```python
from build123d import *

# Parameters (mm, degrees)
SKETCH1_R           = 75
BOSS_EXTRUDE1_DEPTH = 6.35
SKETCH45_R          = 22.1615
SKETCH45_R_2        = 2.0193
CUT_EXTRUDE36_DEPTH = 107.255929246
FILLET2_R           = 10.16


with BuildPart() as part:
    # Sketch1 → Boss-Extrude1 (new body)
    with BuildSketch(Plane(origin=(0, 0, 0), x_dir=(1, 0, 0), z_dir=(0, 1, 0))):
        with Locations(Location((0, 0, 0), (0, 0, 270))):
            Circle(SKETCH1_R)
    extrude(amount=BOSS_EXTRUDE1_DEPTH)

    # Sketch45 → Cut-Extrude36 (cut, through all)
    with BuildSketch(Plane(origin=(0, 6.35, 0), x_dir=(1, 0, 0), z_dir=(0, 1, 0))):
        with Locations(Location((0, 0, 0), (0, 0, 270))):
            Circle(SKETCH45_R)
        with Locations(Location((0, 33.02, 0), (0, 0, 270))):
            Circle(SKETCH45_R_2)
        with Locations(Location((-33.02, 0, 0), (0, 0, 270))):
            Circle(SKETCH45_R_2)
        with Locations(Location((0, -33.02, 0), (0, 0, 270))):
            Circle(SKETCH45_R_2)
        with Locations(Location((33.02, 0, 0), (0, 0, 270))):
            Circle(SKETCH45_R_2)
        with Locations(Location((-25.4, 25.4, 0), (0, 0, 270))):
            Circle(SKETCH45_R_2)
        with BuildLine():
            Line((-32.276051224, 28.683948776), (-54.798637954, 51.206535505))
            ThreePointArc((-54.798637954, 51.206535505), (-54.798637954, 54.798637954), (-51.206535505, 54.798637954))
            Line((-51.206535505, 54.798637954), (-28.683948776, 32.276051224))
            ThreePointArc((-28.683948776, 32.276051224), (-28.683948776, 28.683948776), (-32.276051224, 28.683948776))
        make_face()
        with BuildLine():
            Line((-28.683948776, -32.276051224), (-51.206535505, -54.798637954))
            ThreePointArc((-51.206535505, -54.798637954), (-54.798637954, -54.798637954), (-54.798637954, -51.206535505))
            Line((-54.798637954, -51.206535505), (-32.276051224, -28.683948776))
            ThreePointArc((-32.276051224, -28.683948776), (-28.683948776, -28.683948776), (-28.683948776, -32.276051224))
        make_face()
    extrude(amount=-CUT_EXTRUDE36_DEPTH, mode=Mode.SUBTRACT)

    # Fillet2
    fillet2_edges = [part.edges().sort_by_distance(p)[0] for p in [
        (-51.206535505, 3.175, 54.798637954),
        (-54.798637954, 3.175, 51.206535505),
        (-54.798637954, 3.175, -51.206535505),
        (-51.206535505, 3.175, -54.798637954),
    ]]
    fillet(fillet2_edges, radius=FILLET2_R)


solid = part.part
```
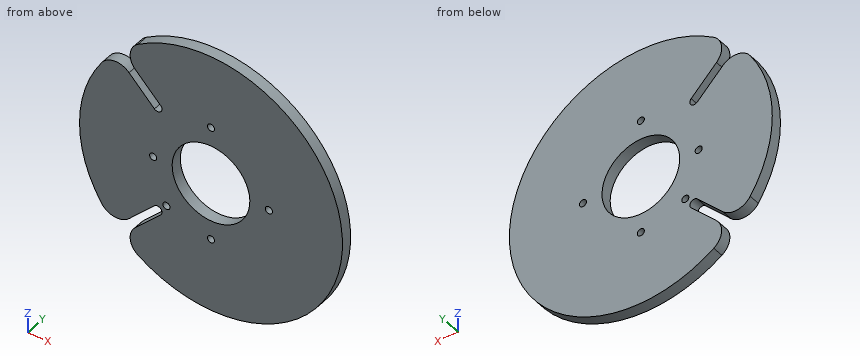
For this review, take the finished solid that the model builds, in its own axes (mm). Give positions to 0.01 mm unless a question says otherwise; leave off trailing zeros. Write each loop counter-clockwise with the first axis right and the second up, starting at its lowest first coordinate (ties: lowest second). Pieces come first, ordered by that corner, then holes. Notation, with made-up numbers: M 26,62 L 60,62 A14 ccw 60,80 Z; hole C 26,89.25 d2. An arc over 180 degrees is marked long. One line per item, written item: value.
1) Take a section at C-C, the plane z = 0. Write out the cut boundary in (x, y), then the cut area to 3 significant figures.
Results are:
outline: M -75,0 L -35.04,0 L -35.04,6.35 L -75,6.35 Z; M -31,0 L -22.16,0 L -22.16,6.35 L -31,6.35 Z; M 22.16,0 L 31,0 L 31,6.35 L 22.16,6.35 Z; M 35.04,0 L 75,0 L 75,6.35 L 35.04,6.35 Z
area: 620 mm²
2) Take a section at A-A, the plane y = 3. Write out the cut boundary in (x, z), then the cut area to 3 significant figures.
Results are:
outline: M -62.39,-41.62 A10.16 ccw -46.76,-43.16 L -32.28,-28.68 A2.54 cw -28.68,-32.28 L -43.16,-46.76 A10.16 ccw -41.62,-62.39 A75 ccw long -41.62,62.39 A10.16 ccw -43.16,46.76 L -28.68,32.28 A2.54 cw -32.28,28.68 L -46.76,43.16 A10.16 ccw -62.39,41.62 A75 ccw Z; hole C -33.02,0 d4.04; hole C -25.4,-25.4 d4.04; hole C 0,0 d44.32; hole C 0,-33.02 d4.04; hole C 0,33.02 d4.04; hole C 33.02,0 d4.04
area: 15,600 mm²
3) Take a section at D-D, the plane x = -25.4. Write out the cut boundary in (y, z), then the cut area to 3 significant figures.
Results are:
outline: M 0,-70.57 L 6.35,-70.57 L 6.35,-27.42 L 0,-27.42 Z; M 0,-23.38 L 6.35,-23.38 L 6.35,70.57 L 0,70.57 Z
area: 871 mm²
4) Take a section at B-B, the plane x = 17.5. Write out the cut boundary in (y, z).
Results are:
outline: M 0,-72.93 L 6.35,-72.93 L 6.35,-13.6 L 0,-13.6 Z; M 0,13.6 L 6.35,13.6 L 6.35,72.93 L 0,72.93 Z
5) For line 1 (Z direction, x = -36, y = 3.5); line 2 (Z direction, x = -16, y = 0.75); line 3 (X direction, y = 1.5, z = -25.4), list the stretches that pass through material, from the lowest coordinate up. Write a range as from..to.
Results are:
line 1: z = -65.8..-39.59, -32.41..32.41, 39.59..65.8
line 2: z = -73.27..-15.33, 15.33..73.27
line 3: x = -70.57..-27.42, -23.38..70.57
6) For P1, Ø1.5, axis at y = 1.5, z = -7, coming from the +X side; P2, Ø3, axis at x = -31, y = 5, coming from the -Z side; P3, Ø3, axis at y = 3.5, z = 41.5, coming from the -X side, all flat-tipped, find the tip position at first contact; note any pin that passes through.
Results are:
P1: stops at x = 74.74
P2: stops at z = -68.95
P3: stops at x = -63.44
